Geometry check sheet. Reference: the model listing, model coordinates, mm. A direction names the side the tool comes from. Round coordinates to 2 decimals unless told otherwise and drop trailing zeros. Order: outer loops, then holes, each group sorted by start corner. A loop starts at its lowest first (then second) coordinate and runs counter-clockwise, first axis right, second up. Notation, with made-up numbers: (87, 71) -> (99, 71) arc R12 ccw to (99, 94) -> close; hole circle Ø6 at (-37, -23). An arc over 180 degrees is marked (long way). Answer as a JSON object with one key per item and string values. Group by question number.
from build123d import *

# Parameters (mm, degrees)
SKETCH1_R           = 1.5
BOSS_EXTRUDE1_DEPTH = 2.5
SKETCH2_R           = 1
CUT_EXTRUDE1_DEPTH  = 10
SKETCH3_R           = 1
CUT_EXTRUDE2_DEPTH  = 10


with BuildPart() as part:
    # Sketch1 → Boss-Extrude1 (new body)
    with BuildSketch(Plane(origin=(0, 0, 0), x_dir=(1, 0, 0), z_dir=(0, 1, 0))):
        Polygon((-36.388124659, -49.061762216), (-46.388124659, -49.061762216), (-46.388124659, -119.061762216), (43.611875341, -119.061762216), (43.611875341, -49.061762216), (33.611875341, -49.061762216), (23.611875341, -28.368941333), (23.611875341, 3.086787883), (49.344702977, -12.442380613), (67.344702977, -12.442380613), (67.344702977, 2.557619387), (28.457213072, 41.451875118), (18.457213072, 41.451875118), (18.457213072, 58.451875118), (-21.230778371, 58.451875118), (-21.230778371, 41.451875118), (-31.230778371, 41.451875118), (-70.125034102, 2.564385214), (-70.125034102, -12.435614786), (-52.125034102, -12.435614786), (-26.388124659, 3.086787883), (-26.388124659, -28.368941333), align=None)
        with Locations(Location((41.111875341, -51.561762216, 0), (0, 0, 270))):
            Circle(SKETCH1_R, mode=Mode.SUBTRACT)
        with Locations(Location((-43.888124659, -51.561762216, 0), (0, 0, 270))):
            Circle(SKETCH1_R, mode=Mode.SUBTRACT)
        with Locations(Location((-43.888124659, -116.561762216, 0), (0, 0, 270))):
            Circle(SKETCH1_R, mode=Mode.SUBTRACT)
        with Locations(Location((41.111875341, -116.561762216, 0), (0, 0, 270))):
            Circle(SKETCH1_R, mode=Mode.SUBTRACT)
    extrude(amount=-BOSS_EXTRUDE1_DEPTH)

    # Sketch2 → Cut-Extrude1 (cut)
    with BuildSketch(Plane(origin=(0, 0, 0), x_dir=(1, 0, 0), z_dir=(0, 1, 0))):
        with Locations(Location((-42.188124659, -87.461762216, 0), (0, 0, 270))):
            Circle(SKETCH2_R)
        with Locations(Location((-42.188124659, -104.561762216, 0), (0, 0, 270))):
            Circle(SKETCH2_R)
    extrude(amount=-CUT_EXTRUDE1_DEPTH, mode=Mode.SUBTRACT)

    # Sketch3 → Cut-Extrude2 (cut)
    with BuildSketch(Plane(origin=(0, 0, 0), x_dir=(1, 0, 0), z_dir=(0, 1, 0))):
        with Locations(Location((39.381875341, -87.461762216, 0), (0, 0, 270))):
            Circle(SKETCH3_R)
        with Locations(Location((39.381875341, -104.561762216, 0), (0, 0, 270))):
            Circle(SKETCH3_R)
    extrude(amount=-CUT_EXTRUDE2_DEPTH, mode=Mode.SUBTRACT)


solid = part.part
Item 1: Thickness scan on L1, parallel to X at y = -0.5, z = 3; L2, parallel to X at y = -1.85, z = 5.5; L3, parallel to Z at x = -22, y = -2.4. Record the ranges inside material, lowest first.
Item 2: Depth check by flat-ended pin: pin 1 Ø0.8 at (x, y) = (25, -1) entering from -Z; pin 2 Ø4 at (x, z) = (-43.89, 116.56) entering from +Y; pin 3 Ø1.2 at (y, z) = (-1, 80) entering from -X; pin 4 Ø1.8 at (x, z) = (39.38, 104.56) entering from +Y (3 decimals). Enter the tip coordinate at first touch or a pass-through.
Item 3: Sectioned sample at C-C, the plane x = -24. Enter the section's corners in (y, z), then the cut area to 3 significant figures.
Item 4: Sectioned sample at D-D, the plane z = 60. Enter the section's corners in (x, y), then the cut area to 3 significant figures.
Item 5: Mould release check, pull along Z, two halves, no side actions. Record for faces 1 (the flat face through (-2, 0, 29)), 2 (the flat face through (48.173, -1.232, -21.732)), 3 (the flat face through (-39.437, -1.232, 4.783)): pulls with the +Z half, pulls with the -Z half, needs draft (parallel to the pull), parting line crosses it, or undercut.
Item 6: Sectioned sample at B-B, the plane y = -1.55. Count the separate pieces of the cut face and the enclosed holes in it, then the cut area to 3 significant figures.
Item 7: Set-up check for faces 4 (the flat face through (-50.406, -1.232, -22.28)), 5 (the flat face through (-31.32, -1.23, 38.57)), 6 (the flat face through (36.3, -1.23, 4.57)), 7 (the flat face through (-2, -2.5, 29)), 8 (the flat face through (28.7, -1.2, 38.9)): record each of +Z, -Z, +X, -X, +Y, -Y from which the full face is reachable in a straight line by a thin tool's end or side.
Item 8: Sectioned sample at A-A, the plane z = 9. Enter the section's corners in (x, y).
Result:
{
 "1": {"L1": "x = -70.13 to -36.48, -26.39 to 23.61, 33.7 to 67.34", "L2": "x = -70.13 to -40.63, -26.39 to 23.61, 37.84 to 67.34", "L3": "z = -41.45 to 119.06"},
 "2": {"pin 1": "stops at z = -41.45", "pin 2": "stops at y = 0", "pin 3": "stops at x = -46.39", "pin 4": "passes through"},
 "3": {"outline": "(-2.5, -41.45) -> (0, -41.45) -> (0, 119.06) -> (-2.5, 119.06) -> close", "area": "401 mm2"},
 "4": {"outline": "(-46.39, -2.5) -> (43.61, -2.5) -> (43.61, 0) -> (-46.39, 0) -> close", "area": "225 mm2"},
 "5": {"face 1": "needs draft", "face 2": "pulls with the -Z half", "face 3": "undercut"},
 "6": {"separate pieces": "1", "enclosed holes": "8", "area": "14,500 mm2"},
 "7": {"face 4": "-Z, -X, +Y, -Y", "face 5": "-X, +Y, -Y", "face 6": "+Y, -Y", "face 7": "+Z, -Z, +X, -X, -Y", "face 8": "+X, +Y, -Y"},
 "8": {"outline": "(-70.13, -2.5) -> (-46.43, -2.5) -> (-46.43, 0) -> (-70.13, 0) -> close; (-26.39, -2.5) -> (23.61, -2.5) -> (23.61, 0) -> (-26.39, 0) -> close; (43.64, -2.5) -> (67.34, -2.5) -> (67.34, 0) -> (43.64, 0) -> close"}
}
